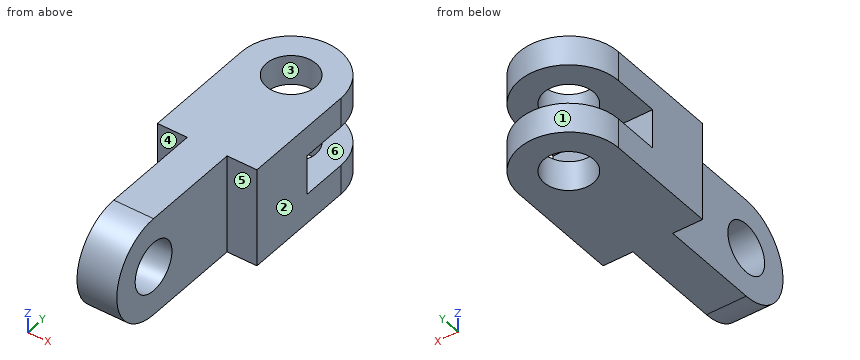
from build123d import *

# Parameters (mm, degrees)
BOSS_EXTRUDE1_DEPTH        = 50
BOSS_EXTRUDE1_DEPTH_BACK   = 50
CUT_EXTRUDE1_DEPTH         = 199.584759445
F_25_0_50_DIAMETER_HOLE1_D = 50
SKETCH7_W                  = 40
SKETCH7_H                  = 50
REVOLVE1_ANGLE             = 180
F_1_0_50_DIAMETER_HOLE1_D  = 50


with BuildPart() as part:
    # Sketch1 → Boss-Extrude1 (new, two sides: drawn at the far end of the back side and taken through both)
    with BuildSketch(Plane.XY.offset(-BOSS_EXTRUDE1_DEPTH_BACK)):
        with BuildLine():
            Line((20, 0), (50, 0))
            Line((50, 0), (50, 114.121621622))
            ThreePointArc((50, 114.121621622), (0, 164.121621622), (-50, 114.121621622))
            Line((-50, 114.121621622), (-50, 0))
            Line((-50, 0), (-20, 0))
            Line((-20, 0), (-20, -100))
            Line((-20, -100), (20, -100))
            Line((20, -100), (20, 0))
        make_face()
    extrude(amount=BOSS_EXTRUDE1_DEPTH + BOSS_EXTRUDE1_DEPTH_BACK)

    # Sketch4 → Cut-Extrude1 (cut, through all)
    with BuildSketch(Plane(origin=(50, 0, 0), x_dir=(0, 0, -1), z_dir=(1, 0, 0))):
        Polygon((-20, 114.121621622), (-20, 67.847884716), (20, 67.847884716), (20, 168.662891807), (-20, 168.662891807), align=None)
    extrude(amount=-CUT_EXTRUDE1_DEPTH, mode=Mode.SUBTRACT)

    # Ø25.0 (50) Diameter Hole1 (through all)
    with Locations(Plane.XY.offset(50)):
        with Locations((0, 114.121621622)):
            Hole(F_25_0_50_DIAMETER_HOLE1_D / 2)

    # Sketch7 → Revolve1 (revolve)
    with BuildSketch(Plane.XZ.offset(100)):
        with Locations((0, 25)):
            Rectangle(SKETCH7_W, SKETCH7_H)
    revolve(axis=Axis((20, -100, 0), (1, 0, 0)), revolution_arc=REVOLVE1_ANGLE)

    # Ø1.0 (50) Diameter Hole1 (through all)
    with Locations(Plane(origin=(20, 0, 0), x_dir=(0, 0, -1), z_dir=(1, 0, 0))):
        with Locations((0, -100)):
            Hole(F_1_0_50_DIAMETER_HOLE1_D / 2)


solid = part.part
Design review of the part built by this model. Coordinates are the model's own, in mm. Face numbers are marked on the shaded views. A direction names the side the tool comes from. Coordinates: 2 decimals unless noted, no trailing zeros. Write each loop counter-clockwise with the first axis right and the second up, starting at its lowest first coordinate (ties: lowest second). Pieces come first, ordered by that corner, then holes. Notation, with made-up numbers: (12, 7.5) - (29, 7.5) arc R28 ccw to (29, 43.5) - close; hole circle Ø2 at (73, 79.25). An arc over 180 degrees is marked (long way). Use one line per item in the form item = value.
Q1. Consider section B-B (z = -14.5). Write out the cut boundary in (x, y), plus the area to 3 significant figures.
Taken from the geometry:
outline = (-50, 0) - (-20, 0) - (-20, -79.63) - (20, -79.63) - (20, 0) - (50, 0) - (50, 67.85) - (-50, 67.85) - close; (-20, -147.85) - (20, -147.85) - (20, -120.37) - (-20, -120.37) - close
area = 11,100 mm^2
Q2. For probe 1 along Y at (x, z) = (3, 0); probe 2 along Z at (x, y) = (-37.5, 91); probe 3 along X at (y, z) = (-69, 43), list the stretches that pass through material, from the lowest coordinate up.
Taken from the geometry:
probe_1 = -150 to -125, -75 to 67.85
probe_2 = -50 to -20, 20 to 50
probe_3 = -20 to 20
Q3. Consider section D-D (z = 34). Write out the cut boundary in (x, y), plus the area to 3 significant figures.
Taken from the geometry:
outline = (-50, 0) - (-20, 0) - (-20, -136.66) - (20, -136.66) - (20, 0) - (50, 0) - (50, 114.12) arc R50 ccw to (-50, 114.12) - close; hole circle Ø50 at (0, 114.12)
area = 18,800 mm^2
Q4. Consider section C-C (y = 123). Write out the cut boundary in (x, z).
Taken from the geometry:
outline = (-49.21, -50) - (-23.37, -50) - (-23.37, -20) - (-49.21, -20) - close; (-49.21, 20) - (-23.37, 20) - (-23.37, 50) - (-49.21, 50) - close; (23.37, -50) - (49.21, -50) - (49.21, -20) - (23.37, -20) - close; (23.37, 20) - (49.21, 20) - (49.21, 50) - (23.37, 50) - close
Q5. Consider section A-A (x = 0). Write out the cut boundary in (y, z), plus the area to 3 significant figures.
Taken from the geometry:
outline = (-100, -50) - (89.12, -50) - (89.12, -20) - (67.85, -20) - (67.85, 20) - (89.12, 20) - (89.12, 50) - (-100, 50) arc R50 ccw to start; (139.12, -50) - (164.12, -50) - (164.12, -20) - (139.12, -20) - close; (139.12, 20) - (164.12, 20) - (164.12, 50) - (139.12, 50) - close; hole circle Ø50 at (-100, 0)
area = 21,500 mm^2
Q6. Insertion check: pin 1 Ø3 at (y, z) = (-63, 5.5) entering from -X; pin 2 Ø1.5 at (x, z) = (32.5, 32.5) entering from -Y; pin 3 Ø6 at (x, z) = (-36, 18) entering from +Y; pin 4 Ø12 at (x, y) = (9, 126.5) entering from -Z. Each pin has a flat end and moves straight along its axis. Give the tip position at first contact, or say it passes through.
Taken from the geometry:
pin_1 = -20
pin_2 = 0
pin_3 = 151
pin_4 = through
Q7. Machinability: for the marked faces 4, 5 and 6, which of the approach directions +Z, -Z, +X, -X, +Y, -Y give a long, thin tool a straight path to every point of the face, cutting with its end or side? Answer none if there is none.
Taken from the geometry:
face_4 = +Z, -Z, -X, -Y
face_5 = +Z, -Z, +X, -Y
face_6 = +X, -X, +Y
Q8. The part is to be moulded in two halves that separate along X. For the marked faces 1, 2 and 3, say which applies: +X half, -X half, draft (parallel to the pull), parting line (faces both ways), or undercut.
Taken from the geometry:
face_1 = parting line
face_2 = +X half
face_3 = undercut
